Input: part model. Units: mm. Frame: model coordinates. A direction names the side the tool comes from. Give positions to 0.01 mm unless a question says otherwise; leave off trailing zeros. Order: outer loops, then holes, each group sorted by start corner. A loop starts at its lowest first (then second) coordinate and runs counter-clockwise, first axis right, second up.
```python
from build123d import *

# Parameters (mm, degrees)
F0_W = 5
F0_H = 5


with BuildPart() as f1:
    # F0 (on Front) → F1 (revolve)
    with BuildSketch(Plane.XZ):
        Polygon((-5, 0), (0, 0), (0, 5), (-70.414929, 5), (-127.732546, 85.890315), (-143.274711, 85.890315), (-133.327724, 75.321652), (-126.371749, 75.321652), (-73, 0), align=None)
        with Locations((-2.5, -2.5)):
            Rectangle(F0_W, F0_H)
    revolve(axis=Axis((0, 0, 191.825941), (0, 0, 1)))


solid = f1.part
```
1) Pull-direction query (Y, two-part tool) for faces 1 (the face through (1.08, 4.88, -2.46)), 2 (the face through (-1, -1, 5)), 3 (the face through (-15, -1, 0)); classes: pulls with the +Y half, pulls with the -Y half, needs draft (parallel to the pull), parting line crosses it, or undercut.
2) First-contact query: P1, Ø1.5, axis at y = 23, z = 44.5, coming from the -X side; P2, Ø10, axis at y = 74, z = 49.5, coming from the +X side; P3, Ø3, axis at y = -13, z = 21.5, coming from the -X side. Flat tips, straight axial feed; report the tip coordinate or a pass-through.
3) Line query: probe 1 along X at (y, z) = (-35.5, 70); probe 2 along X at (y, z) = (-63, 44.5); probe 3 along Z at (x, y) = (59.5, 27). Output: solid intervals per line, ascending.
4) Cut plane D-D (z = 10.5). Return the cut outline in (x, y), then the cut area to 3 significant figures.
5) Cut plane A-A (y = 0). Return the cut outline in (x, z).
6) Reachability of faces 4 (the face through (0, 0, -5)), 5 (the face through (-118, 49, 75.322)) from +Z, -Z, +X, -X, +Y, -Y: full face, straight path, thin tool, end or side. Return the list, or none.
7) Cut plane C-C (z = 47). Return the cut outline in (x, y).
Geometry says:
1. face 1: parting line crosses it
1. face 2: undercut
1. face 3: needs draft
2. P1: stops at x = -102.54
2. P2: stops at x = 85.23
2. P3: stops at x = -88.37
3. probe 1: x = -117.35 to -110.93, 110.93 to 117.35
3. probe 2: x = -83.41 to -75.59, 75.59 to 83.41
3. probe 3: z = 0 to 5
4. outline: circle Ø160.88 at (0, 0); hole circle Ø148.62 at (0, 0)
4. area: 2,980 mm2
5. outline: (-143.27, 85.89) - (-133.33, 75.32) - (-126.37, 75.32) - (-73, 0) - (-5, 0) - (-5, -5) - (5, -5) - (5, 0) - (73, 0) - (126.37, 75.32) - (133.33, 75.32) - (143.27, 85.89) - (127.73, 85.89) - (70.41, 5) - (-70.41, 5) - (-127.73, 85.89) - close
6. face 4: -Z, +X, -X, +Y, -Y
6. face 5: -Z
7. outline: circle Ø212.61 at (0, 0); hole circle Ø200.35 at (0, 0)
